Here's how the part is built. I have some questions about the finished solid (model axes, mm). Coordinates: 2 decimals unless noted, no trailing zeros. Write each loop counter-clockwise with the first axis right and the second up, starting at its lowest first coordinate (ties: lowest second). Pieces come first, ordered by that corner, then holes.
(1) For pin 1 Ø1.9 at (x, z) = (4.5, -2) entering from -Y; pin 2 Ø3 at (x, y) = (2, 30.5) entering from +Z; pin 3 Ø1.9 at (x, y) = (2.5, 236) entering from -Z, each with a flat end and sliding along its axis, tell me the tip position at first contact or that it passes through.
(2) Imagine slicing it at A-A, the plane z = 96. List the corners of the cut face in (x, y) for me, plus the area to 3 significant figures.
(3) Please list where these lines run through material, in increasing order: probe 1 along Y at (x, z) = (2.75, -19.05); probe 2 along Z at (x, y) = (5.75, 122).
(4) Imagine slicing it at B-B, the plane x = 4. State how many separate pieces and enclosed holes the cut face has, plus the area to 3 significant figures.
```python
from build123d import *

# Parameters (mm, degrees)
SKETCH1_R           = 1.75
BOSS_EXTRUDE1_DEPTH = 6.35
SKETCH2_W           = 12.7
SKETCH2_H           = 6.35
CUT_EXTRUDE1_DEPTH  = 7.35
LPATTERN1_COUNT     = 10
LPATTERN1_PITCH     = 25.4
SKETCH3_W           = 6.35
SKETCH3_H           = 12.7
CUT_EXTRUDE2_DEPTH  = 7.35
LPATTERN2_COUNT     = 10
LPATTERN2_PITCH     = 25.4
SKETCH4_W           = 6.35
SKETCH4_H           = 12.7
CUT_EXTRUDE3_DEPTH  = 7.35
SKETCH5_W           = 12.7
SKETCH5_H           = 6.35
CUT_EXTRUDE4_DEPTH  = 7.35
LPATTERN3_COUNT     = 5
LPATTERN3_PITCH     = 25.4
SKETCH6_W           = 6.35
SKETCH6_H           = 12.7
CUT_EXTRUDE5_DEPTH  = 7.35
LPATTERN4_COUNT     = 8
LPATTERN4_PITCH     = 25.4
SKETCH7_W           = 12.7
SKETCH7_H           = 6.35
CUT_EXTRUDE6_DEPTH  = 7.35
SKETCH8_W           = 6.35
SKETCH8_H           = 6.35
CUT_EXTRUDE7_DEPTH  = 7.35
SKETCH9_R           = 3.96875
CUT_EXTRUDE8_DEPTH  = 7.35
SKETCH10_R          = 12.7
CUT_EXTRUDE9_DEPTH  = 7.35


with BuildPart() as part:
    # Sketch1 → Boss-Extrude1 (new body)
    with BuildSketch(Plane(origin=(0, 0, 0), x_dir=(0, 0, -1), z_dir=(1, 0, 0))):
        Polygon((0, 0), (0, 190.5), (-127, 190.5), (-127, 254), (114.3, 254), (114.3, 0), align=None)
        with Locations((-107.95, 234.95)):
            Circle(SKETCH1_R, mode=Mode.SUBTRACT)
        with Locations((-107.95, 209.55)):
            Circle(SKETCH1_R, mode=Mode.SUBTRACT)
        with Locations((19.05, 234.95)):
            Circle(SKETCH1_R, mode=Mode.SUBTRACT)
        with Locations((95.25, 234.95)):
            Circle(SKETCH1_R, mode=Mode.SUBTRACT)
        with Locations((19.05, 19.05)):
            Circle(SKETCH1_R, mode=Mode.SUBTRACT)
        with Locations((95.25, 19.05)):
            Circle(SKETCH1_R, mode=Mode.SUBTRACT)
    extrude(amount=BOSS_EXTRUDE1_DEPTH)

    # Sketch2 → Cut-Extrude1 (cut, through all)
    with BuildSketch(Plane(origin=(6.35, 0, 0), x_dir=(0, 0, -1), z_dir=(1, 0, 0))):
        with Locations((-107.95, 250.825)):
            Rectangle(SKETCH2_W, SKETCH2_H)
    cut_extrude1 = extrude(amount=-CUT_EXTRUDE1_DEPTH, mode=Mode.SUBTRACT)

    # LPattern1: Cut-Extrude1 ×10
    with Locations(*[(0, 0, -i * LPATTERN1_PITCH) for i in range(1, LPATTERN1_COUNT)]):
        add(cut_extrude1, mode=Mode.SUBTRACT)

    # Sketch3 → Cut-Extrude2 (cut, through all)
    with BuildSketch(Plane(origin=(6.35, 0, 0), x_dir=(0, 0, -1), z_dir=(1, 0, 0))):
        with Locations((111.125, 234.95)):
            Rectangle(SKETCH3_W, SKETCH3_H)
    cut_extrude2 = extrude(amount=-CUT_EXTRUDE2_DEPTH, mode=Mode.SUBTRACT)

    # LPattern2: Cut-Extrude2 ×10
    with Locations(*[(0, -i * LPATTERN2_PITCH, 0) for i in range(1, LPATTERN2_COUNT)]):
        add(cut_extrude2, mode=Mode.SUBTRACT)

    # Sketch4 → Cut-Extrude3 (cut, through all)
    with BuildSketch(Plane(origin=(6.35, 0, 0), x_dir=(0, 0, -1), z_dir=(1, 0, 0))):
        with Locations((-123.825, 234.95)):
            Rectangle(SKETCH4_W, SKETCH4_H)
        with Locations((-123.825, 209.55)):
            Rectangle(SKETCH4_W, SKETCH4_H)
    extrude(amount=-CUT_EXTRUDE3_DEPTH, mode=Mode.SUBTRACT)

    # Sketch5 → Cut-Extrude4 (cut, through all)
    with BuildSketch(Plane(origin=(6.35, 0, 0), x_dir=(0, 0, -1), z_dir=(1, 0, 0))):
        with Locations((-107.95, 193.675)):
            Rectangle(SKETCH5_W, SKETCH5_H)
    cut_extrude4 = extrude(amount=-CUT_EXTRUDE4_DEPTH, mode=Mode.SUBTRACT)

    # LPattern3: Cut-Extrude4 ×5
    with Locations(*[(0, 0, -i * LPATTERN3_PITCH) for i in range(1, LPATTERN3_COUNT)]):
        add(cut_extrude4, mode=Mode.SUBTRACT)

    # Sketch6 → Cut-Extrude5 (cut, through all)
    with BuildSketch(Plane(origin=(6.35, 0, 0), x_dir=(0, 0, -1), z_dir=(1, 0, 0))):
        with Locations((3.175, 6.35)):
            Rectangle(SKETCH6_W, SKETCH6_H)
    cut_extrude5 = extrude(amount=-CUT_EXTRUDE5_DEPTH, mode=Mode.SUBTRACT)

    # LPattern4: Cut-Extrude5 ×8
    with Locations(*[(0, i * LPATTERN4_PITCH, 0) for i in range(1, LPATTERN4_COUNT)]):
        add(cut_extrude5, mode=Mode.SUBTRACT)

    # Sketch7 → Cut-Extrude6 (cut, through all)
    with BuildSketch(Plane(origin=(6.35, 0, 0), x_dir=(0, 0, -1), z_dir=(1, 0, 0))):
        with Locations((19.05, 3.175)):
            Rectangle(SKETCH7_W, SKETCH7_H)
        with Locations((44.45, 3.175)):
            Rectangle(SKETCH7_W, SKETCH7_H)
        with Locations((69.85, 3.175)):
            Rectangle(SKETCH7_W, SKETCH7_H)
        with Locations((95.25, 3.175)):
            Rectangle(SKETCH7_W, SKETCH7_H)
    extrude(amount=-CUT_EXTRUDE6_DEPTH, mode=Mode.SUBTRACT)

    # Sketch8 → Cut-Extrude7 (cut, through all)
    with BuildSketch(Plane(origin=(6.35, 0, 0), x_dir=(0, 0, -1), z_dir=(1, 0, 0))):
        with Locations((9.525, 3.175)):
            Rectangle(SKETCH8_W, SKETCH8_H)
        with Locations((104.775, 3.175)):
            Rectangle(SKETCH8_W, SKETCH8_H)
    extrude(amount=-CUT_EXTRUDE7_DEPTH, mode=Mode.SUBTRACT)

    # Sketch9 → Cut-Extrude8 (cut, through all)
    with BuildSketch(Plane(origin=(6.35, 0, 0), x_dir=(0, 0, -1), z_dir=(1, 0, 0))):
        with Locations((-88.9, 222.25)):
            Circle(SKETCH9_R)
    extrude(amount=-CUT_EXTRUDE8_DEPTH, mode=Mode.SUBTRACT)

    # Sketch10 → Cut-Extrude9 (cut, through all)
    with BuildSketch(Plane(origin=(6.35, 0, 0), x_dir=(0, 0, -1), z_dir=(1, 0, 0))):
        with Locations((-38.1, 222.25)):
            Circle(SKETCH10_R)
    extrude(amount=-CUT_EXTRUDE9_DEPTH, mode=Mode.SUBTRACT)


solid = part.part
```
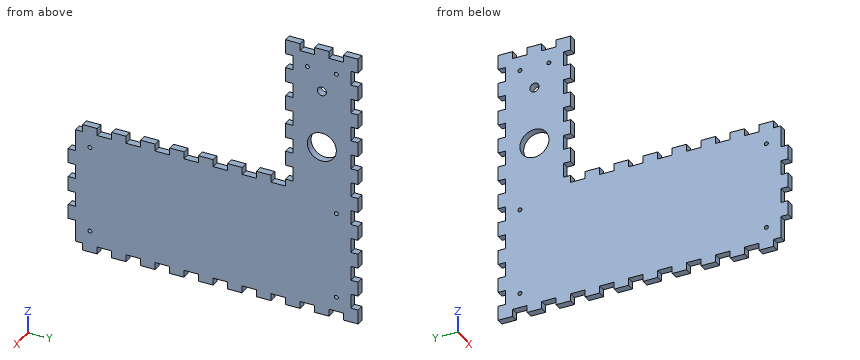
Recorded:
1. pin 1: stops at y = 12.7
1. pin 2: stops at z = -6.35
1. pin 3: stops at z = -107.95
2. outline: (0, 190.5) - (6.35, 190.5) - (6.35, 254) - (0, 254) - close
2. area: 403 mm2
3. probe 1: y = 6.35 to 17.3, 20.8 to 233.2, 236.7 to 247.65
3. probe 2: z = -114.3 to 0
4. separate pieces: 1
4. enclosed holes: 8
4. area: 33,300 mm2
